For this review, use the dimensioned drawing (mm, ordinates from the lowest corner) and the shaded views. A direction names the side the tool comes from. Coordinates: 2 decimals unless noted, no trailing zeros. Loops run counter-clockwise (first coordinate to the right, second up) from the corner with the lowest first, then second, coordinate; pieces in that order, holes last. Notation, with made-up numbers: M 57.25,-8.75 L 97.25,-8.75 A9 ccw 97.25,-0.75 Z; hole C 86.25,5.5 d11. An arc over 180 degrees is marked long. Write item = value, one per line.
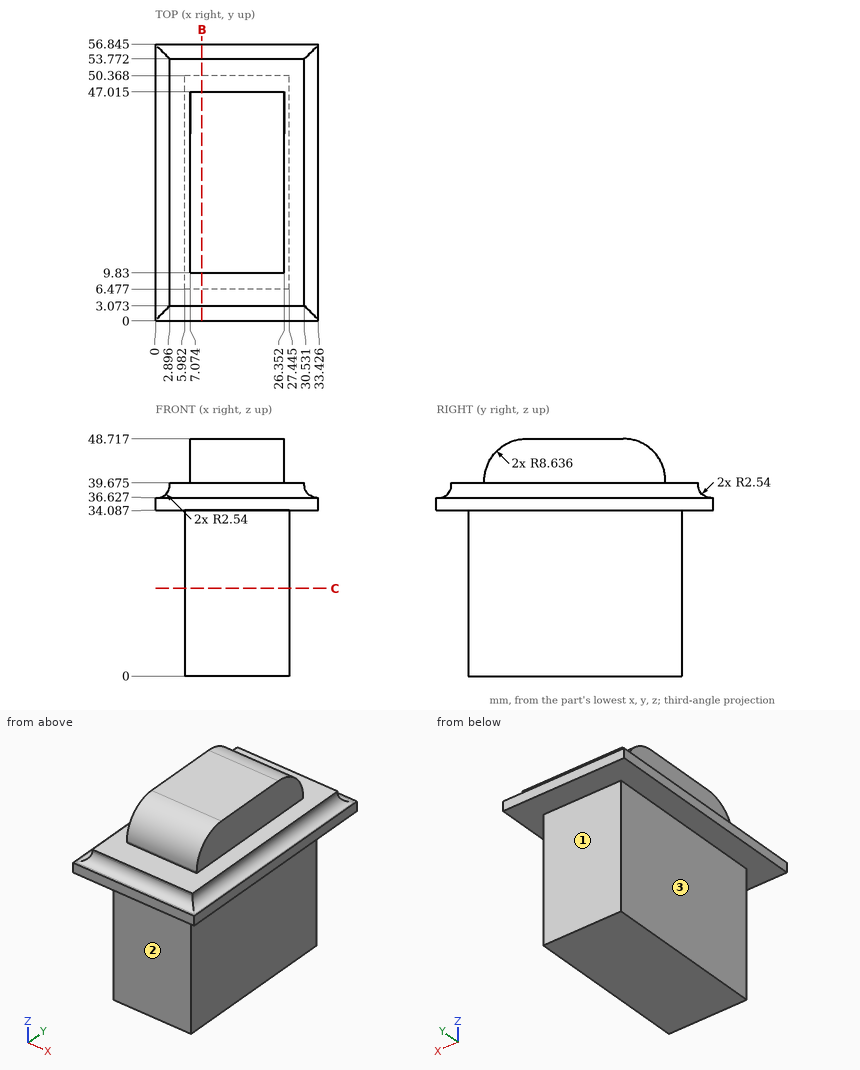
Q1. Machinability: for the marked faces 1, 2 and 3, which of the approach directions +Z, -Z, +X, -X, +Y, -Y give a long, thin tool a straight path to every point of the face, cutting with its end or side? Answer none if there is none.
Solved:
face_1 = -Z, +X, -X, +Y
face_2 = -Z, +X, -X, -Y
face_3 = -Z, -X, +Y, -Y
Q2. For pin 1 Ø8 at (x, y) = (9.5, 7.5) entering from -Z; pin 2 Ø4 at (x, y) = (12, 9) entering from +Z (1 decimal); pin 3 Ø17 at (x, z) = (20.5, 18.5) entering from +Y; pin 4 Ø10 at (y, z) = (30, 45.5) entering from +X, all flat-tipped, find the tip position at first contact; note any pin that passes through.
Solved:
pin_1 = 0
pin_2 = 44.4
pin_3 = 50.37
pin_4 = 26.35
Q3. Add section C-C (z = 18). Write out the cut boundary in (x, y) (1 decimal), and give its area (3 significant figures).
Solved:
outline = M 6,6.5 L 27.4,6.5 L 27.4,50.4 L 6,50.4 Z
area = 942 mm²
Q4. For line 1 along X through (y, z) = (32, 44); line 2 along X through (y, z) = (46.5, 26) (1 decimal); line 3 along Y through (x, z) = (15.5, 28), list the stretches that pass through material, from the lowest coordinate up.
Solved:
line_1 = 7.07 to 26.35
line_2 = 6 to 27.4
line_3 = 6.48 to 50.37
Q5. Add section B-B (x = 9.5). Write out the cut boundary in (y, z) (1 decimal).
Solved:
outline = M 0,34.1 L 6.5,34.1 L 6.5,0 L 50.4,0 L 50.4,34.1 L 56.8,34.1 L 56.8,36.6 L 56.3,36.6 A2.5 cw 53.8,39.2 L 53.8,39.7 L 47,39.7 L 47,40.1 A8.6 ccw 38.4,48.7 L 18.5,48.7 A8.6 ccw 9.8,40.1 L 9.8,39.7 L 3.1,39.7 L 3.1,39.2 A2.5 cw 0.5,36.6 L 0,36.6 Z
